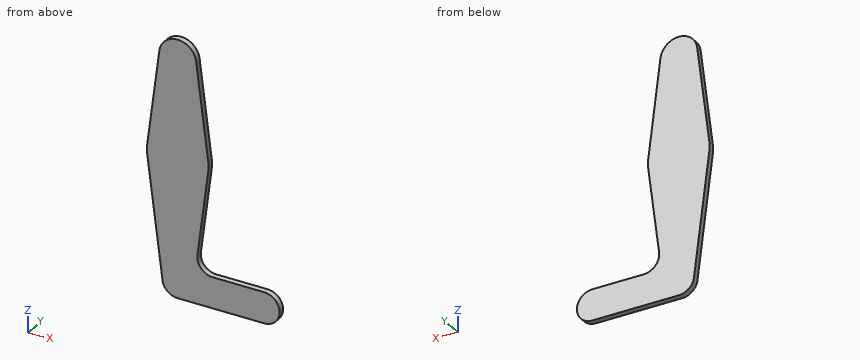
```python
from build123d import *

# Parameters (mm, degrees)
F0_R     = 3.175
F1_DEPTH = 3.048


# Not quite as in the source:
# - ends of sketch curves that miss each other by under 0.0002 mm in the source are joined


with BuildPart() as f1:
    # F0 (on Front) → F1 (new body)
    with BuildSketch(Plane.XZ):
        with BuildLine():
            ThreePointArc((-7.9375, 0), (0, 7.9375), (7.9375, 0))
            ThreePointArc((7.9375, 0), (5.6126600757, -5.6126600757), (0, -7.9375))
            Line((0, -7.9375), (44.45, -7.9375))
            ThreePointArc((44.45, -7.9375), (36.5125, 0), (44.45, 7.9375))
            Line((44.45, 7.9375), (18.0149584735, 7.9375))
            ThreePointArc((18.0149584735, 7.9375), (12.0523084735, 10.6291369817), (10.127113946, 16.881475))
            Line((10.127113946, 16.881475), (15.7504882737, 61.515625))
            ThreePointArc((15.7504882737, 61.515625), (15.8438414904, 62.5058612634), (15.875, 63.5))
            ThreePointArc((15.875, 63.5), (15.8438414904, 64.4941387366), (15.7504882737, 65.484375))
            ThreePointArc((15.7504882737, 65.484375), (0, 79.375), (-15.7504882737, 65.484375))
            ThreePointArc((-15.7504882737, 65.484375), (-15.875, 63.4999684915), (-15.7504803964, 61.5155624772))
            Line((-15.7504803964, 61.5155624772), (-7.9375, 0))
        make_face()
        with Locations((0, 63.5)):
            Circle(F0_R, mode=Mode.SUBTRACT)
        with BuildLine():
            Line((-9.4502929642, 115.490625), (-15.7504882737, 65.484375))
            ThreePointArc((-15.7504882737, 65.484375), (0, 79.375), (15.7504882737, 65.484375))
            Line((15.7504882737, 65.484375), (9.4502929642, 115.490625))
            ThreePointArc((9.4502929642, 115.490625), (9.5063048942, 114.896483242), (9.525, 114.3))
            ThreePointArc((9.525, 114.3), (-0.596483242, 104.7936951058), (-9.4502929642, 115.490625))
        make_face()
        with Locations((-3.175, 100.0252)):
            Circle(F0_R, mode=Mode.SUBTRACT)
        with BuildLine():
            ThreePointArc((9.4502929642, 115.490625), (0, 123.825), (-9.4502929642, 115.490625))
            ThreePointArc((-9.4502929642, 115.490625), (-0.596483242, 104.7936951058), (9.525, 114.3))
            ThreePointArc((9.525, 114.3), (9.5063048942, 114.896483242), (9.4502929642, 115.490625))
        make_face()
        with Locations((0, 114.3)):
            Circle(F0_R, mode=Mode.SUBTRACT)
        with BuildLine():
            ThreePointArc((0, -7.9375), (5.6126600757, -5.6126600757), (7.9375, 0))
            ThreePointArc((7.9375, 0), (0, 7.9375), (-7.9375, 0))
            ThreePointArc((-7.9375, 0), (-5.6126600757, -5.6126600757), (0, -7.9375))
        make_face()
        Circle(F0_R, mode=Mode.SUBTRACT)
        with BuildLine():
            ThreePointArc((44.45, 7.9375), (36.5125, 0), (44.45, -7.9375))
            ThreePointArc((44.45, -7.9375), (50.0626600757, -5.6126600757), (52.3875, 0))
            ThreePointArc((52.3875, 0), (50.0626600757, 5.6126600757), (44.45, 7.9375))
        make_face()
        with Locations((44.45, 0)):
            Circle(F0_R, mode=Mode.SUBTRACT)
        with Locations((44.45, 0)):
            Circle(F0_R)
        with Locations((0, 63.5)):
            Circle(F0_R)
        with Locations((-3.175, 100.0252)):
            Circle(F0_R)
        with Locations((0, 114.3)):
            Circle(F0_R)
        Circle(F0_R)
    extrude(amount=F1_DEPTH)


solid = f1.part
```
Work out the finished part from the listing and answer in its coordinate system (mm). Give positions to 0.01 mm unless a question says otherwise; leave off trailing zeros. Loops run counter-clockwise (first coordinate to the right, second up) from the corner with the lowest first, then second, coordinate; pieces in that order, holes last. Notation, with made-up numbers: (47, 66) -> (81, 66) arc R11 ccw to (81, 77) -> close; hole circle Ø4 at (-32.75, -17). An arc over 180 degrees is marked (long way). One line per question, with ' | ' between items. Start each with the question number.
1) Section C-C, the plane x = 32 is taken. Determine the outline of the cut face in (y, z), then the cut area to 3 significant figures.
2) Section B-B, the plane x = 13.5 is taken. Determine the outline of the cut face in (y, z).
3) Section D-D, the plane z = 36.5 is taken. Determine the outline of the cut face in (x, y).
4) This flat-tipped pin is pushed along its axis until it touches: pin 1 (0.9 mm diameter, centred on x = 29.5, y = -1.5, fed in from +Z). Where does it stop, or does it pass through?
5) Straight lines are drawn through the part: L1, parallel to X at y = -0.95, z = -0.5; L2, parallel to Z at x = 22, y = -0.45; L3, parallel to Z at x = 0, y = -2.6 (1 decimal). For each, find the intervals that lie inside material, in ascending order.
Resolved:
1) outline: (-3.05, -7.94) -> (0, -7.94) -> (0, 7.94) -> (-3.05, 7.94) -> close | area: 48.4 mm2
2) outline: (-3.05, -7.94) -> (0, -7.94) -> (0, 9.34) -> (-3.05, 9.34) -> close; (-3.05, 43.65) -> (0, 43.65) -> (0, 83.35) -> (-3.05, 83.35) -> close
3) outline: (-12.57, -3.05) -> (12.6, -3.05) -> (12.6, 0) -> (-12.57, 0) -> close
4) pin 1: z = 7.94
5) L1: -7.92 to 52.37 | L2: -7.94 to 7.94 | L3: -7.9 to 123.8
